```python
from build123d import *

# Parameters (mm, degrees)
F1_DEPTH       = 35
F3_D           = 5
F3_START       = 1.8205079
F3_CBORE_D     = 10
F3_CBORE_DEPTH = 8


with BuildPart() as f1:
    # F0 (on Top) → F1 (new body, symmetric)
    with BuildSketch(Plane.XY):
        with BuildLine():
            ThreePointArc((-17.3192642082, 2.5086026559), (17.5, 0), (-17.3192642082, -2.5086026559))
            Line((-17.3192642082, -2.5086026559), (-28.1192642082, -2.5086026559))
            Line((-28.1192642082, -2.5086026559), (-28.1192642082, -10.9086026559))
            ThreePointArc((-28.1192642082, -10.9086026559), (-25.7761184577, -16.5654569054), (-20.1192642082, -18.9086026559))
            Line((-20.1192642082, -18.9086026559), (-7.9192642082, -18.9086026559))
            ThreePointArc((-7.9192642082, -18.9086026559), (20.5, 0), (-7.9192642082, 18.9086026559))
            Line((-7.9192642082, 18.9086026559), (-20.1192642082, 18.9086026559))
            ThreePointArc((-20.1192642082, 18.9086026559), (-25.7761184577, 16.5654569054), (-28.1192642082, 10.9086026559))
            Line((-28.1192642082, 10.9086026559), (-28.1192642082, 2.5086026559))
            Line((-28.1192642082, 2.5086026559), (-17.3192642082, 2.5086026559))
        make_face()
    extrude(amount=F1_DEPTH, both=True)

    # F3 (through all)
    # its depths count from where the whole tool has entered the part; down to there all is cleared
    with Locations(Plane(origin=(0, 18.9086026559, 0), x_dir=(-1, 0, 0), z_dir=(0, 1, 0)).offset(-F3_START)):
        with Locations((20.2, 22.25), (20.2, 7.25), (20.2, -8.25), (20.2, -24.25)):
            CounterBoreHole(F3_D / 2, F3_CBORE_D / 2, F3_CBORE_DEPTH)


solid = f1.part
```
The model under review builds one solid part; all positions refer to its coordinate system, in mm. A direction names the side the tool comes from. Round coordinates to 2 decimals unless told otherwise and drop trailing zeros. Write each loop counter-clockwise with the first axis right and the second up, starting at its lowest first coordinate (ties: lowest second). Pieces come first, ordered by that corner, then holes. Notation, with made-up numbers: (2.25, 8.25) - (57.25, 8.25) arc R10 cw to (57.25, 17.25) - close; hole circle Ø10 at (79.25, -34.75). An arc over 180 degrees is marked (long way). Answer as CSV lines item,"result". Start each with the question number.
(1) For pin 1 Ø8 at (x, z) = (-20.2, -24.25) entering from +Y; pin 2 Ø6 at (x, z) = (-20, 1) entering from -Y; pin 3 Ø8.5 at (x, z) = (-23.5, 14) entering from +Y, all flat-tipped, find the tip position at first contact; note any pin that passes through.
(2) For faces 4 (the flat face through (-15, 9.4, 35)), 5 (the flat face through (-23, -2.509, 0)), 6 (the cylindrical face through (-16.23, 14.07, 19.21)), list the 3-axis set-ups (+Z, -Z, +X, -X, +Y, -Y) from which the entire face can be reached by the end or side of a thin tool; tool diameter is ignored.
(3) Draft analysis for pull direction Y (two halves, no side actions). For faces 1 (the flat face through (-28.119, -7, 0)), 2 (the flat face through (-23, 2.509, 0)), 3 (the flat face through (-13, 18.909, 0)), state which applies: pulls with the +Y half, pulls with the -Y half, needs draft (parallel to the pull), parting line crosses it, or undercut.
(4) We need section A-A on x = 0. State the section outline as (y, z) points.
(5) We need section D-D on y = 10. State the section outline as (x, z) points, plus the area to 3 significant figures.
(6) We need section C-C on z = -24.25. State the section outline as (x, y) points.
(7) To check wall thickness, follow line 1 (Z direction, x = -20.2, y = 13.25); line 2 (Z direction, x = -20.2, y = -9.5); line 3 (X direction, y = -16, z = 9). State the ranges of each line that lie inside material, in increasing order.
(8) We need section B-B on y = -15.5. State the section outline as (x, z) points, plus the area to 3 significant figures.
Worked answers:
1,pin 1,"y = 9.09"
1,pin 2,"y = -18.91"
1,pin 3,"y = 18.91"
2,face 4,"+Z, +X, -X, +Y, -Y"
2,face 5,"+Z, -Z, -X"
2,face 6,"+Y"
3,face 1,"needs draft"
3,face 2,"undercut"
3,face 3,"pulls with the +Y half"
4,outline,"(-20.5, -35) - (-17.5, -35) - (-17.5, 35) - (-20.5, 35) - close; (17.5, -35) - (20.5, -35) - (20.5, 35) - (17.5, 35) - close"
5,outline,"(-28.12, -35) - (-14.36, -35) - (-14.36, 35) - (-28.12, 35) - close; (14.36, -35) - (17.9, -35) - (17.9, 35) - (14.36, 35) - close; hole circle Ø10 at (-20.2, -24.25); hole circle Ø10 at (-20.2, -8.25); hole circle Ø10 at (-20.2, 7.25); hole circle Ø10 at (-20.2, 22.25)"
5,area,"896 mm²"
6,outline,"(-28.12, -10.91) arc R8 ccw to (-22.7, -18.48) - (-22.7, -2.51) - (-28.12, -2.51) - close; (-28.12, 2.51) - (-22.7, 2.51) - (-22.7, 9.09) - (-25.2, 9.09) - (-25.2, 17.09) arc R8 ccw to (-28.12, 10.91) - close; (-17.7, -18.91) - (-7.92, -18.91) arc R20.5 ccw (long way) to (-7.92, 18.91) - (-15.2, 18.91) - (-15.2, 9.09) - (-17.7, 9.09) - (-17.7, 2.51) - (-17.32, 2.51) arc R17.5 cw (long way) to (-17.32, -2.51) - (-17.7, -2.51) - close"
7,line 1,"-35 to -29.25, -19.25 to -13.25, -3.25 to 2.25, 12.25 to 17.25, 27.25 to 35"
7,line 2,"-35 to -26.75, -21.75 to -10.75, -5.75 to 4.75, 9.75 to 19.75, 24.75 to 35"
7,line 3,"-26.29 to -21.99, -18.41 to -7.09, 7.09 to 12.82"
8,outline,"(-26.67, -35) - (-8.12, -35) - (-8.12, 35) - (-26.67, 35) - close; (8.12, -35) - (13.42, -35) - (13.42, 35) - (8.12, 35) - close; hole circle Ø5 at (-20.2, -24.25); hole circle Ø5 at (-20.2, -8.25); hole circle Ø5 at (-20.2, 7.25); hole circle Ø5 at (-20.2, 22.25)"
8,area,"1,590 mm²"
